Can you work these out from the model? Positions are in its coordinate system, mm. A direction names the side the tool comes from. Coordinates: 2 decimals unless noted, no trailing zeros. Loops run counter-clockwise (first coordinate to the right, second up) from the corner with the lowest first, then second, coordinate; pieces in that order, holes last. Notation, with made-up numbers: M -21.75,-32 L -11.75,-32 A33 ccw -11.75,-3 Z; hole C -12.75,-6.5 d7. An arc over 180 degrees is marked long. Answer as a JSON object with one key per item and string values. Group by question number.
Item 1: Suppose I cut it at C-C (x = 6.75). Write out the boundary of the cut face in (y, z) (3 decimals).
Item 2: I'm going to push flat-ended pins straight in: pin 1 Ø4 at (x, y) = (9, 1) entering from -Z (3 decimals); pin 2 Ø1 at (x, y) = (9, 2) entering from +Z; pin 3 Ø3 at (x, z) = (7, 2.5) entering from +Y. Where does each tip first touch, or does it pass through?
Item 3: If I drill on line 1 (X direction, y = 1, z = 4); line 2 (X direction, y = -1.75, z = -1.5); line 3 (Z direction, x = 3, y = 3), over which ranges is the centre line in solid material (lowest first)?
Item 4: Suppose I cut it at A-A (x = 1.75). Write out the boundary of the cut face in (y, z) (1 decimal), then the cut area to 3 significant figures.
Item 5: Which directions (+Z, -Z, +X, -X, +Y, -Y) give clear straight access to the entire face, cutting with the end or side of a thin tool? Please do faces 1 (the cylindrical face through (2.66, 1.03, -4.65)), 2 (the cylindrical face through (8, -1.5, -2.8)), 3 (the flat face through (0.99, 0.86, -0.51)).
Item 6: Suppose I cut it at B-B (x = 3.5). Write out the boundary of the cut face in (y, z) (1 decimal), then the cut area to 3 significant figures.
Item 7: We'd pull the mould along Z, two halves only. Please class faces 4 (the flat face through (11.112, -1.4, -1.4)), 5 (the flat face through (1, 0, -1)), 6 (the flat face through (0.99, 0.87, 0.49)), 7 (the cylindrical face through (13.27, -0.73, -1.41)): +Z half, -Z half, draft (parallel to the pull), parting line (faces both ways), or undercut.
```python
from build123d import *

# Parameters (mm, degrees)
CUT_EXTRUDE1_DEPTH = 2


with BuildPart() as part:
    # Sketch1 → Revolve1 (revolve)
    with BuildSketch(Plane.XY, mode=Mode.PRIVATE) as revolve1_sk:
        Polygon((0, 0), (0, 4.2625), (0.5, 4.7625), (4.7625, 4.7625), (4.7625, 3.175), (11.1125, 3.175), (11.1125, 1.5875), (15.375, 1.5875), (15.875, 1.0875), (15.875, 0), align=None)
    revolve(revolve1_sk.sketch.rotate(Axis((15.875, 0, 0), (-1, 0, 0)), 180), axis=Axis((15.875, 0, 0), (-1, 0, 0)))

    # Sketch2 → Cut-Revolve1 (revolve, cut)
    with BuildSketch(Plane.XY, mode=Mode.PRIVATE) as cut_revolve1_sk:
        Polygon((0, 0), (0, 1), (2, 1), (2.577350269, 0), align=None)
    revolve(cut_revolve1_sk.sketch.rotate(Axis((2.577350269, 0, 0), (-1, 0, 0)), 180), axis=Axis((2.577350269, 0, 0), (-1, 0, 0)), mode=Mode.SUBTRACT)

    # Sketch3 → Cut-Extrude1 (cut)
    with BuildSketch(Plane(origin=(0, 0, 0), x_dir=(0, 0, -1), z_dir=(1, 0, 0))):
        Polygon((-1, 0.577350269), (-1, -0.577350269), (0, -1.154700538), (1, -0.577350269), (1, 0.577350269), (0, 1.154700538), align=None)
    extrude(amount=CUT_EXTRUDE1_DEPTH, mode=Mode.SUBTRACT)


solid = part.part
```
From the geometry:
{
 "1": {"outline": "C 0,0 d6.35"},
 "2": {"pin 1": "z = -3.175", "pin 2": "z = 2.8", "pin 3": "y = 3.01"},
 "3": {"line 1": "0 to 4.76", "line 2": "0 to 11.11", "line 3": "-3.7 to 3.7"},
 "4": {"outline": "C 0,0 d9.5; hole M -1.2,0 L -0.6,-1 L 0.6,-1 L 1.2,0 L 0.6,1 L -0.6,1 Z", "area": "67.8 mm2"},
 "5": {"face 1": "+X, -X", "face 2": "+X", "face 3": "-X"},
 "6": {"outline": "C 0,0 d9.5", "area": "71.3 mm2"},
 "7": {"face 4": "draft", "face 5": "undercut", "face 6": "undercut", "face 7": "parting line"}
}
